from build123d import *

# Parameters (mm, degrees)
EXTRUDE_1_DEPTH = 30
FILLET_1_R      = 30
SKETCH_2_R      = 15
EXTRUDE_2_DEPTH = 25
SHELL_1_T       = -2
FILLET_3_R      = 5
FILLET_4_R      = 1


with BuildPart() as part:
    # 草图1 → 凸台-拉伸1 (new, symmetric)
    with BuildSketch(Plane.XY):
        with BuildLine():
            Line((60, 100), (-60, 100))
            Line((-60, 100), (-65.899969295, -68.953015099))
            ThreePointArc((-65.899969295, -68.953015099), (-57.498438495, -90.839751114), (-35.918244485, -100))
            Line((-35.918244485, -100), (35.918244485, -100))
            ThreePointArc((35.918244485, -100), (57.498438495, -90.839751114), (65.899969295, -68.953015099))
            Line((65.899969295, -68.953015099), (60, 100))
        make_face()
    extrude(amount=EXTRUDE_1_DEPTH, both=True)

    # 圆角1
    fillet_1_edges = [part.edges().sort_by_distance(p)[0] for p in [
        (-60, 100, 0),
        (60, 100, 0),
    ]]
    fillet(fillet_1_edges, radius=FILLET_1_R)

    # 草图2 → 凸台-拉伸2 (add)
    with BuildSketch(Plane(origin=(0, 100, 0), x_dir=(1, 0, 0), z_dir=(0, 1, 0))):
        Circle(SKETCH_2_R)
    extrude(amount=EXTRUDE_2_DEPTH)

    # 抽壳1
    shell_1_openings = [part.faces().sort_by_distance(p)[0] for p in [
        (0, 125, 0),
    ]]
    offset(amount=SHELL_1_T, openings=shell_1_openings, kind=Kind.INTERSECTION)

    # 圆角3
    fillet_3_edges = [part.edges().sort_by_distance(p)[0] for p in [
        (0, -100, 30),
        (57.498438495, -90.839751114, 30),
        (0, 100, -30),
        (0, 100, 30),
        (63.455515431, 1.046984901, 30),
        (-63.455515431, 1.046984901, -30),
        (-51.86908787, 91.58019401, -30),
        (51.86908787, 91.58019401, -30),
        (-63.455515431, 1.046984901, 30),
        (-51.86908787, 91.58019401, 30),
        (51.86908787, 91.58019401, 30),
        (-15, 100, 0),
        (63.455515431, 1.046984901, -30),
        (57.498438495, -90.839751114, -30),
        (0, -100, -30),
        (-57.498438495, -90.839751114, -30),
        (-57.498438495, -90.839751114, 30),
    ]]
    fillet(fillet_3_edges, radius=FILLET_3_R)

    # 圆角4
    fillet_4_edges = [part.edges().sort_by_distance(p)[0] for p in [
        (-15, 125, 0),
        (-13, 125, 0),
    ]]
    fillet(fillet_4_edges, radius=FILLET_4_R - 0.0001)  # a hair under: the kernel refuses the full size


solid = part.part
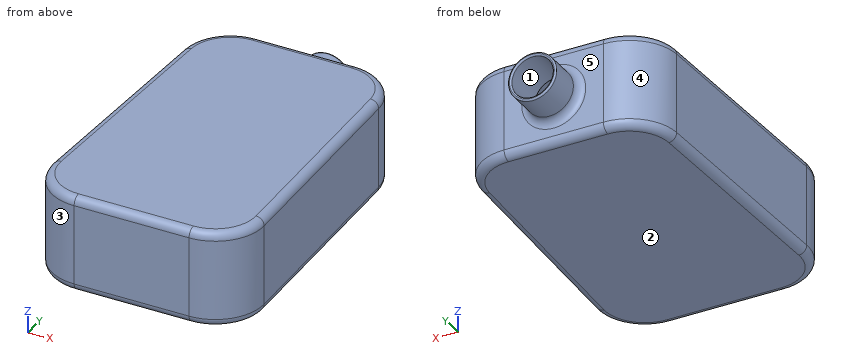
CAD build for the part. Positions are in the model's coordinates, mm. Face numbers are marked on the shaded views. A direction names the side the tool comes from. Give positions to 0.01 mm unless a question says otherwise; leave off trailing zeros. Write each loop counter-clockwise with the first axis right and the second up, starting at its lowest first coordinate (ties: lowest second). Pieces come first, ordered by that corner, then holes. Notation, with made-up numbers: (10.5, 69.5) -> (36.5, 69.5) arc R25 ccw to (36.5, 83.5) -> close; hole circle Ø2 at (7, -27). An arc over 180 degrees is marked (long way). Return JSON: item names as keys, results as strings.
Item 1: Band-saw the part on A-A (x = 26). List the corners of the cut face in (y, z), then the cut area to 3 significant figures.
Answer below:
{"outline": "(-100, -25) arc R5 ccw to (-95, -30) -> (95, -30) arc R5 ccw to (100, -25) -> (100, 25) arc R5 ccw to (95, 30) -> (-95, 30) arc R5 ccw to (-100, 25) -> close; hole (-98, -28) -> (98, -28) -> (98, 28) -> (-98, 28) -> close", "area": "1,000 mm2"}
Item 2: Drop flat-ended pins along their axis: pin 1 (5 mm diameter, centred on x = 6.5, z = 3.5, fed in from +Y); pin 2 (10 mm diameter, centred on x = -37.5, z = 9.5, fed in from +Y). Give the stop position or say it passes through.
Answer below:
{"pin 1": "stops at y = -98", "pin 2": "stops at y = 99.96"}
Item 3: Drill centre lines: probe 1 along Z at (x, y) = (38, 82); probe 2 along Y at (x, z) = (-27, 10.5); probe 3 along Z at (x, y) = (0, 107). Where is each one in solid material? Low to high.
Answer below:
{"probe 1": "z = -30 to -28, 28 to 30", "probe 2": "y = -100 to -98, 98 to 100", "probe 3": "z = -15 to -13, 13 to 15"}
Item 4: Two-plate mould, pull along Z, no slides. Class the marked faces 1, 2 and 3: +Z half, -Z half, draft (parallel to the pull), parting line (faces both ways), or undercut.
Answer below:
{"face 1": "undercut", "face 2": "-Z half", "face 3": "draft"}
Item 5: Tool access for the marked faces 4 and 5: list every direction of +Z, -Z, +X, -X, +Y, -Y with a clear straight run to the whole face (end or side of a thin tool).
Answer below:
{"face 4": "+Z, -Z, -X, +Y", "face 5": "+Y"}
